Part model, mm, in its own coordinate system. A direction names the side the tool comes from. Give positions to 0.01 mm unless a question says otherwise; leave off trailing zeros. Order: outer loops, then holes, each group sorted by start corner. A loop starts at its lowest first (then second) coordinate and runs counter-clockwise, first axis right, second up. Notation, with made-up numbers: (30, 46) - (85, 46) arc R21 ccw to (85, 84) - close; hole circle Ø2 at (29, -6). An arc over 180 degrees is marked (long way). One line per item, written item: value.
Autodesk Inventor part; units mm, degrees
ref_plane "YZ Plane" through (0, 0, 0) normal (1, 0, 0) x (0, 1, 0)
ref_plane "XZ Plane" through (0, 0, 0) normal (0, 1, 0) x (-1, 0, 0)
ref_plane "XY Plane" through (0, 0, 0) normal (0, 0, 1) x (1, 0, 0)
sketch "Sketch2" plane through (0, 0, 0) normal (0, 0, 1) x (1, 0, 0)
  line L0 (-6, 2.6) -> (6, 2.6)
  line L1 (6, 2.6) -> (6, -2.6)
  line L2 (6, -2.6) -> (-6, -2.6)
  line L3 (-6, -2.6) -> (-6, 2.6)
  line L4 (-7.2, 3) -> (7.2, 3)
  line L5 (7.2, 3) -> (7.2, -3)
  line L6 (7.2, -3) -> (-7.2, -3)
  line L7 (-7.2, -3) -> (-7.2, 3)
  point P0 (0, 0)
  point P1 (0, 2.6)
  point P2 (-6, 0)
  point P3 (-7.2, 0)
  point P4 (0, 3)
  dimension "d0" = 5.2
  dimension "d1" = 12
  dimension "d23" = 6
  dimension "d24" = 14.4
extrude "Extrusion1" add sketch "Sketch2" along normal mid plane 14.4 contours L0 L1 L2 L3 | L4 L5 L6 L7
sketch "Sketch3" plane through (0, 0, 7.2) normal (0, 0, 1) x (1, 0, 0)
  line L0 (-4.8, 1.158) -> (4.8, 1.158)
  line L1 (4.8, 1.158) -> (4.8, -0.442)
  line L2 (4.8, -0.442) -> (-4.8, -0.442)
  line L3 (-4.8, -0.442) -> (-4.8, 1.158)
  line L4 (-6, 2.6) -> (6, 2.6)
  line L5 (-6, -2.6) -> (-6, 2.6)
  line L6 (6, -2.6) -> (-6, -2.6)
  line L7 (6, 2.6) -> (6, -2.6)
  point P0 (0, 0)
  point P1 (0, -0.442)
  dimension "d4" = 1.6
  dimension "d5" = 9.6
  dimension "d25" = 0.442
extrude "Extrusion2" cut sketch "Sketch3" against normal blind 13.6
extrude "Extrusion3" cut sketch "Sketch3" against normal blind 0.8 contours L0 L1 L2 L3
chamfer "Chamfer1" distance 0.4 angle 45 4 edges at (-4.8, 0.358, 6.4) (0, 1.158, 6.4) (0, -0.442, 6.4) (4.8, 0.358, 6.4)
sketch "Sketch4" plane through (-4.8, -0.442, -6.4) normal (0, -1, 0) x (1, 0, 0)
  line L0 (0, 0) -> (9.6, 0)
  line L1 (0.4, 11.58) -> (2, 11.58)
  line L2 (2, 11.58) -> (2, 0)
  line L3 (2, 0) -> (0.4, 0)
  line L4 (0.4, 0) -> (0.4, 11.58)
  line L5 (2.8, 11.58) -> (4.4, 11.58)
  line L6 (4.4, 11.58) -> (4.4, 0)
  line L7 (4.4, 0) -> (2.8, 0)
  line L8 (2.8, 0) -> (2.8, 11.58)
  line L9 (5.2, 11.58) -> (6.8, 11.58)
  line L10 (6.8, 11.58) -> (6.8, 0)
  line L11 (6.8, 0) -> (5.2, 0)
  line L12 (5.2, 0) -> (5.2, 11.58)
  line L13 (7.6, 11.58) -> (9.2, 11.58)
  line L14 (9.2, 11.58) -> (9.2, 0)
  line L15 (9.2, 0) -> (7.6, 0)
  line L16 (7.6, 0) -> (7.6, 11.58)
  line L17 (2, 11.58) -> (2.8, 11.58) construction
  line L18 (4.4, 11.58) -> (5.2, 11.58) construction
  line L19 (6.8, 11.58) -> (7.6, 11.58) construction
  point P0 (4.8, 6.4)
  point P1 (4.8, 11.58)
  dimension "d18" = 11.58
  dimension "d19" = 1.6
  dimension "d20" = 0.8
extrude "Extrusion4" add sketch "Sketch4" along normal blind 0.001
equation "\"d4\" = wall"
properties part number "11032-Black" material "ABS Plastic"
1) Cut at A-A, the plane z = 3. Give the number of separate pieces and of enclosed holes in the cut face, then the cut area to 3 significant figures.
Outcome:
separate pieces: 2
enclosed holes: 1
area: 39.4 mm^2
2) Cut at C-C, the plane y = -1.8. Give the cut face in (x, z).
Outcome:
outline: (-7.2, -7.2) - (7.2, -7.2) - (7.2, 7.2) - (6, 7.2) - (6, -6.4) - (-6, -6.4) - (-6, 7.2) - (-7.2, 7.2) - close
3) Mould opens along Y. For faces 3 (the flat face through (0, 3, 0)), 4 (the flat face through (-4, -0.443, -1)), 5 (the flat face through (0, 0, -7.2)) say: released by +Y, released by -Y, zero draft, split by the parting line, or undercut.
Outcome:
face 3: released by +Y
face 4: undercut
face 5: zero draft
4) Drill centre lines: line 1 along Y through (x, z) = (-3.5, 0.5); line 2 along X through (y, z) = (-0.4, 4); line 3 along Y through (x, z) = (-5.25, -6). Where is each one in solid material? Low to high. Write a range as from..to.
Outcome:
line 1: y = -3..-2.6, -0.44..1.16, 2.6..3
line 2: x = -7.2..-6, -4.8..4.8, 6..7.2
line 3: y = -3..-2.6, 2.6..3
5) Which spindle directions (+Z, -Z, +X, -X, +Y, -Y) get a long thin tool onto all of the face, cutting with end or side? Do faces 1 (the flat face through (1, -0.443, -1)), 2 (the flat face through (0, -3, 0)). Say none if no direction does.
Outcome:
face 1: +Z
face 2: +Z, -Z, +X, -X, -Y
6) Cut at D-D, the plane x = 0. Give the cut face in (y, z).
Outcome:
outline: (-3, -7.2) - (3, -7.2) - (3, 7.2) - (2.6, 7.2) - (2.6, -6.4) - (1.16, -6.4) - (1.16, 6) - (0.76, 6.4) - (-0.04, 6.4) - (-0.44, 6) - (-0.44, -6.4) - (-2.6, -6.4) - (-2.6, 7.2) - (-3, 7.2) - close
